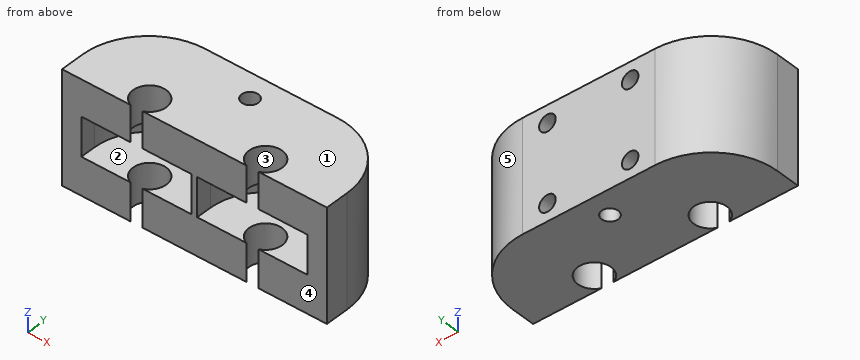
from build123d import *

# Parameters (mm, degrees)
SKETCH1_W           = 48
SKETCH1_H           = 20.3
BOSS_EXTRUDE1_DEPTH = 16.3
SKETCH2_R           = 3
CUT_EXTRUDE1_DEPTH  = 55.605677361
CUT_EXTRUDE2_DEPTH  = 3.5
FILLET1_R           = 12
SKETCH4_R           = 1.5
CUT_EXTRUDE3_DEPTH  = 55.605677361
SKETCH5_R           = 1.5
CUT_EXTRUDE4_DEPTH  = 8


with BuildPart() as part:
    # Sketch1 → Boss-Extrude1 (new body)
    with BuildSketch(Plane(origin=(0, 0, 0), x_dir=(1, 0, 0), z_dir=(0, 1, 0))):
        with Locations((24, -10.15)):
            Rectangle(SKETCH1_W, SKETCH1_H)
    extrude(amount=BOSS_EXTRUDE1_DEPTH)

    # Sketch2 → Cut-Extrude1 (cut, through all)
    with BuildSketch(Plane.XY.offset(20.3)):
        with Locations((13.5, 2.8)):
            Circle(SKETCH2_R)
        with Locations((34.5, 2.8)):
            Circle(SKETCH2_R)
    extrude(amount=-CUT_EXTRUDE1_DEPTH, mode=Mode.SUBTRACT)

    # Sketch3 → Cut-Extrude2 (cut, symmetric)
    with BuildSketch(Plane.XY.offset(10.3)):
        with BuildLine():
            Line((3.5, 2.8), (3.5, -6.25))
            Line((3.5, -6.25), (23.495503035, -6.25))
            Line((23.495503035, -6.25), (23.495503035, 3.099865091))
            ThreePointArc((23.495503035, 3.099865091), (13.350050596, 12.798875696), (3.5, 2.8))
        make_face()
        with BuildLine():
            Line((24.5, 2.8), (24.5, -6.25))
            Line((24.5, -6.25), (44.495503035, -6.25))
            Line((44.495503035, -6.25), (44.495503035, 3.099865091))
            ThreePointArc((44.495503035, 3.099865091), (34.350050596, 12.798875696), (24.5, 2.8))
        make_face()
    extrude(amount=CUT_EXTRUDE2_DEPTH, both=True, mode=Mode.SUBTRACT)

    # Fillet1
    fillet1_edges = [part.edges().sort_by_distance(p)[0] for p in [
        (48, 16.3, 10.15),
        (0, 16.3, 10.15),
    ]]
    fillet(fillet1_edges, radius=FILLET1_R)

    # Sketch4 → Cut-Extrude3 (cut, through all)
    with BuildSketch(Plane(origin=(0, 0, 0), x_dir=(-1, 0, 0), z_dir=(0, 0, -1))):
        with Locations((-24, 11.8)):
            Circle(SKETCH4_R)
    extrude(amount=-CUT_EXTRUDE3_DEPTH, mode=Mode.SUBTRACT)

    # Sketch5 → Cut-Extrude4 (cut)
    with BuildSketch(Plane(origin=(0, 16.3, 0), x_dir=(1, 0, 0), z_dir=(0, 1, 0))):
        with Locations(Location((31.5, -17.15, 0), (0, 0, 270))):
            Circle(SKETCH5_R)
        with Locations(Location((16.5, -17.15, 0), (0, 0, 270))):
            Circle(SKETCH5_R)
        with Locations(Location((16.5, -3.15, 0), (0, 0, 270))):
            Circle(SKETCH5_R)
        with Locations(Location((31.5, -3.15, 0), (0, 0, 270))):
            Circle(SKETCH5_R)
    extrude(amount=-CUT_EXTRUDE4_DEPTH, mode=Mode.SUBTRACT)


solid = part.part
Build history of the part. All positions in model axes, mm. Face numbers are marked on the shaded views. A direction names the side the tool comes from. Coordinates: 2 decimals unless noted, no trailing zeros. Write each loop counter-clockwise with the first axis right and the second up, starting at its lowest first coordinate (ties: lowest second). Pieces come first, ordered by that corner, then holes. Notation, with made-up numbers: (73, -6.5) -> (125, -6.5) arc R30 cw to (125, 25.5) -> close; hole circle Ø7 at (-12, -28.75). An arc over 180 degrees is marked (long way). Use CSV: the item, a comma, the result in double quotes. Start each with the question number.
Q1. Cut at A-A, the plane z = 14.25. List the corners of the cut face in (x, y), then the cut area to 3 significant figures.
Q2. Cut at D-D, the plane z = 3.15. List the corners of the cut face in (x, y).
Q3. Drill centre lines: probe 1 along X at (y, z) = (2.8, 3.25); probe 2 along Z at (x, y) = (26, 7); probe 3 along X at (y, z) = (14, 3.15). Where is each one in solid material? Low to high.
Q4. Cut at C-C, the plane x = 34.5. List the corners of the cut face in (y, z), then the cut area to 3 significant figures.
Q5. Flat gauge pins, fed straight in: pin 1 Ø4 at (x, y) = (14.5, 5) entering from -Z; pin 2 Ø0.9 at (x, z) = (16.5, 17) entering from +Y; pin 3 Ø1.5 at (x, z) = (5.5, 10) entering from -Y; pin 4 Ø4 at (y, z) = (10, 5) entering from +X. Where does each tip first touch, or does it go through?
Q6. Pull direction Y, two halves, no side cores. Call the marked faces 3, 4 and 5: released by +Y, released by -Y, zero draft, split by the parting line, or undercut.
Q7. 3-axis set-ups, long thin cutter, end or side, ignore diameter. For the marked faces 1 and 2: which of +Z, -Z, +X, -X, +Y, -Y reach the whole face in a straight line?
Q8. Cut at B-B, the plane x = 24. List the corners of the cut face in (y, z).
Checked values:
1,outline,"(0, 0) -> (12.42, 0) arc R3 cw (long way) to (14.58, 0) -> (33.42, 0) arc R3 cw (long way) to (35.58, 0) -> (48, 0) -> (48, 4.3) arc R12 ccw to (36, 16.3) -> (12, 16.3) arc R12 ccw to (0, 4.3) -> close; hole circle Ø3 at (24, 11.8)"
1,area,"658 mm²"
2,outline,"(0, 0) -> (12.42, 0) arc R3 cw (long way) to (14.58, 0) -> (33.42, 0) arc R3 cw (long way) to (35.58, 0) -> (48, 0) -> (48, 4.3) arc R12 ccw to (36, 16.3) -> (33, 16.3) -> (33, 8.3) -> (30, 8.3) -> (30, 16.3) -> (18, 16.3) -> (18, 8.3) -> (15, 8.3) -> (15, 16.3) -> (12, 16.3) arc R12 ccw to (0, 4.3) -> close; hole circle Ø3 at (24, 11.8)"
3,probe 1,"x = 0 to 10.5, 16.5 to 31.5, 37.5 to 48"
3,probe 2,"z = 0 to 6.8, 13.8 to 20.3"
3,probe 3,"x = 4.94 to 15, 18 to 30, 33 to 43.06"
4,outline,"(5.8, 0) -> (16.3, 0) -> (16.3, 20.3) -> (5.8, 20.3) -> (5.8, 13.8) -> (12.8, 13.8) -> (12.8, 6.8) -> (5.8, 6.8) -> close"
4,area,"164 mm²"
5,pin 1,"stops at z = 0"
5,pin 2,"stops at y = 8.3"
5,pin 3,"stops at y = 7.64"
5,pin 4,"stops at x = 47.42"
6,face 3,"undercut"
6,face 4,"released by -Y"
6,face 5,"released by +Y"
7,face 1,"+Z, +X, -X, +Y, -Y"
7,face 2,"-Y"
8,outline,"(0, 0) -> (10.3, 0) -> (10.3, 20.3) -> (0, 20.3) -> close; (13.3, 0) -> (16.3, 0) -> (16.3, 20.3) -> (13.3, 20.3) -> close"
